The listing builds one solid part. Answer for the finished solid, in the listing's coordinates (mm). A direction names the side the tool comes from. Give positions to 0.01 mm unless a question says otherwise; leave off trailing zeros. Order: outer loops, then holes, each group sorted by start corner. A loop starts at its lowest first (then second) coordinate and runs counter-clockwise, first axis right, second up. Notation, with made-up numbers: (52, 75.25) - (67, 75.25) arc R36 cw to (67, 109.25) - close; hole circle Ø6 at (57, 56). An arc over 180 degrees is marked (long way). Use a Markdown table: item, result. Add a question column.
1) Flat-ended cylindrical pins translate along their axes: pin 1 (0.6 mm diameter, centred on y = -12, z = 1, fed in from -X); pin 2 (2 mm diameter, centred on x = 0, z = 2, fed in from +Y); pin 3 (1.9 mm diameter, centred on y = 16, z = -1.5, fed in from +X); pin 4 (4 mm diameter, centred on y = -8, z = 0, fed in from -X). Find the tip coordinate at first contact, or state that the pin passes through.
2) Find section A-A, the plane y = 8. Determine the outline of the cut face in (x, z).
3) Find section C-C, the plane z = 0. State how many separate pieces and enclosed holes the cut face has, plus the area to 3 significant figures.
4) Find section B-B, the plane x = 0.4. Determine the outline of the cut face in (y, z), plus the area to 3 significant figures.
5) Straight lines are drawn through the part: line 1 (Y direction, x = -0.45, z = 0); line 2 (Y direction, x = 0.65, z = 2); line 3 (X direction, y = -11.5, z = -2). For each, find the intervals that lie inside material, in ascending order.
6) For faces 3 (the face through (-1.606, -12.876, 0.694)), 4 (the face through (1.606, 4.876, 0.694)), 5 (the face through (0.017, 1.29, 2.024)), determine the directions among +Z, -Z, +X, -X, +Y, -Y from which every point of the face is accessible in a straight line to the end or side of a thin tool.
7) The mould has two halves that part along Y. Classify faces 1 (the face through (-2, -2, -3)), 2 (the face through (-1.2, 12, 0)): released by +Y, released by -Y, zero draft, split by the parting line, or undercut.
8) Find section D-D, the plane y = -10. Determine the outline of the cut face in (x, z).
Autodesk Inventor part; units mm, degrees
ref_plane "YZ Plane" through (0, 0, 0) normal (1, 0, 0) x (0, 1, 0)
ref_plane "XZ Plane" through (0, 0, 0) normal (0, 1, 0) x (-1, 0, 0)
ref_plane "XY Plane" through (0, 0, 0) normal (0, 0, 1) x (1, 0, 0)
sketch "Sketch3" plane through (0, 0, 0) normal (1, 0, 0) x (0, 1, 0)
  arc A0 (16, -3.6) -> (16, 3.6) centre (16, 0) ccw
  line L0 (-16, -3.6) -> (16, -3.6)
  line L1 (-16, 3.6) -> (16, 3.6)
  arc A1 (-16, 3.6) -> (-16, -3.6) centre (-16, 0) ccw
  line L2 (0, -3.6) -> (0, 3.6) construction
  circle A2 centre (-8, 0) radius 3.2
  circle A3 centre (0, 0) radius 3.2
  line L3 (0, 0) -> (-8, 0) construction
  line L4 (-8, 0) -> (-16, 0) construction
  circle A4 centre (-8, 0) radius 2.4
  circle A5 centre (0, 0) radius 2.4
  circle A6 centre (-16, 0) radius 3.2
  circle A7 centre (-16, 0) radius 2.4
  circle A8 centre (8, 0) radius 3.2
  circle A9 centre (8, 0) radius 2.4
  circle A10 centre (16, 0) radius 3.2
  circle A11 centre (16, 0) radius 2.4
  line L5 (0, 0) -> (8, 0) construction
  line L6 (8, 0) -> (16, 0) construction
  dimension "d49" = 7.2
  dimension "d59" = 6.4
  dimension "d60" = 4.8
  dimension "d64" = 8
extrude "Extrusion4" add sketch "Sketch3" along normal mid plane 4 contours L0 A1 L1 A0 | A2 | A3 | A6 | A8 | A10
sketch "Sketch11" plane through (2, 0, 0) normal (1, 0, 0) x (0, 0, -1)
  circle A0 centre (0, 0) radius 2.4
  circle A1 centre (0, -8) radius 2.4
  circle A2 centre (0, 0) radius 3.2
  circle A3 centre (0, -8) radius 3.2
  circle A4 centre (0, 8) radius 2.4
  arc A5 (3.6, 16) -> (-3.6, 16) centre (0, 16) ccw
  arc A6 (-3.6, -16) -> (3.6, -16) centre (0, -16) ccw
  circle A7 centre (0, -16) radius 3.2
  circle A8 centre (0, 8) radius 3.2
  circle A9 centre (0, 16) radius 3.2
  circle A10 centre (0, 16) radius 2.4
  line L0 (3.6, 16) -> (3.6, -16)
  line L1 (-3.6, -16) -> (-3.6, 16)
  line L2 (-2.5456, 13.4544) -> (-2.5456, 10.5456)
  line L3 (2.5456, 13.4544) -> (2.5456, 10.5456)
  arc A11 (-2.5456, 13.4544) -> (2.5456, 13.4544) centre (0, 16) ccw
  arc A12 (2.5456, 10.5456) -> (-2.5456, 10.5456) centre (0, 8) ccw
  line L4 (0, 16) -> (-2.5456, 13.4544) construction
  line L5 (-2.5456, 5.4544) -> (-2.5456, 2.5456)
  line L6 (2.5456, 5.4544) -> (2.5456, 2.5456)
  arc A13 (-2.5456, 5.4544) -> (2.5456, 5.4544) centre (0, 8) ccw
  arc A14 (2.5456, 2.5456) -> (-2.5456, 2.5456) centre (0, 0) ccw
  line L7 (-2.5456, -2.5456) -> (-2.5456, -5.4544)
  line L8 (2.5456, -2.5456) -> (2.5456, -5.4544)
  arc A15 (-2.5456, -2.5456) -> (2.5456, -2.5456) centre (0, 0) ccw
  arc A16 (2.5456, -5.4544) -> (-2.5456, -5.4544) centre (0, -8) ccw
  line L9 (-2.5456, -10.5456) -> (-2.5456, -13.4544)
  line L10 (2.5456, -10.5456) -> (2.5456, -13.4544)
  arc A17 (-2.5456, -10.5456) -> (2.5456, -10.5456) centre (0, -8) ccw
  arc A18 (2.5456, -13.4544) -> (-2.5456, -13.4544) centre (0, -16) ccw
  dimension "d61" = 6.4
  dimension "d65" = 45
  dimension "d68" = 8
extrude "Extrusion16" cut sketch "Sketch11" against normal blind 0.8 contours A0 | A1 | A2 | A3 | A4 | A7 | A8 | A9 | A10
extrude "Extrusion17" cut sketch "Sketch11" against normal blind 0.8 contours A11 L3 A12 L2 | A13 L6 A14 L5 | A15 L8 A16 L7 | A17 L10 A18 L9
mirror "Mirror3" about plane through (0, 0, 0) normal (1, 0, 0) of "Extrusion16", "Extrusion17"
fillet "Fillet1" radius 0.1 6 edges at (-2, 19.6, 0) (-2, 0, 3.6) (-2, 0, -3.6) (2, 0, 3.6) (2, 0, -3.6) (2, 19.6, 0)
fillet "Fillet1" radius 0.4 32 edges at (1.6, -13.4544, -2.5456) (1.6, -10.5456, -2.5456) (1.6, -10.5456, 2.5456) (1.6, -13.4544, 2.5456) (1.6, -5.4544, 2.5456) (1.6, -2.5456, 2.5456) (1.6, -2.5456, -2.5456) (1.6, -5.4544, -2.5456) (1.6, 2.5456, 2.5456) (1.6, 5.4544, 2.5456) (1.6, 5.4544, -2.5456) (1.6, 2.5456, -2.5456) (1.6, 10.5456, 2.5456) (1.6, 13.4544, 2.5456) (1.6, 13.4544, -2.5456) (1.6, 10.5456, -2.5456) (-1.6, -10.5456, -2.5456) (-1.6, -13.4544, -2.5456) (-1.6, -10.5456, 2.5456) (-1.6, -13.4544, 2.5456) (-1.6, -2.5456, 2.5456) (-1.6, -5.4544, 2.5456) (-1.6, -5.4544, -2.5456) (-1.6, -2.5456, -2.5456) (-1.6, 2.5456, -2.5456) (-1.6, 5.4544, -2.5456) (-1.6, 5.4544, 2.5456) (-1.6, 2.5456, 2.5456) (-1.6, 13.4544, 2.5456) (-1.6, 10.5456, 2.5456) (-1.6, 13.4544, -2.5456) (-1.6, 10.5456, -2.5456)
equation "\"d49\" = tlad"
equation "\"d59\" = tsd"
equation "\"d60\" = tpd"
equation "\"d64\" = lu"
equation "\"d15\" = 0.5 * lu"
equation "\"d61\" = tsd"
equation "\"d68\" = lu"
equation "\"d62\" = tsl"
equation "\"d73\" = 0.5 * lu - 2 * wall"
equation "\"d56\" = lf"
equation "\"d75\" = tf"
properties part number "32017-DKBluishGray" material "ABS Plastic"
The answers:
| question | item | result |
|---|---|---|
| 1 | pin 1 | x = -1.2 |
| 1 | pin 2 | y = 19.46 |
| 1 | pin 3 | x = 1.2 |
| 1 | pin 4 | through |
| 2 | outline | (-2, -3.5) arc R0.1 ccw to (-1.9, -3.6) - (1.9, -3.6) arc R0.1 ccw to (2, -3.5) - (2, -3.2) - (1.2, -3.2) - (1.2, -2.4) - (-1.2, -2.4) - (-1.2, -3.2) - (-2, -3.2) - close; (-2, 3.2) - (-1.2, 3.2) - (-1.2, 2.4) - (1.2, 2.4) - (1.2, 3.2) - (2, 3.2) - (2, 3.5) arc R0.1 ccw to (1.9, 3.6) - (-1.9, 3.6) arc R0.1 ccw to (-2, 3.5) - close |
| 3 | separate pieces | 6 |
| 3 | enclosed holes | 0 |
| 3 | area | 42.9 mm2 |
| 4 | outline | (-16, -3.6) - (16, -3.6) arc R3.6 ccw to (16, 3.6) - (-16, 3.6) arc R3.6 ccw to start; hole circle Ø4.8 at (-16, 0); hole circle Ø4.8 at (-8, 0); hole circle Ø4.8 at (0, 0); hole circle Ø4.8 at (8, 0); hole circle Ø4.8 at (16, 0) |
| 4 | area | 181 mm2 |
| 5 | line 1 | -19.6 to -18.4, -13.6 to -10.4, -5.6 to -2.4, 2.4 to 5.6, 10.4 to 13.6, 18.4 to 19.6 |
| 5 | line 2 | -18.99 to -17.33, -14.67 to -9.33, -6.67 to -1.33, 1.33 to 6.67, 9.33 to 14.67, 17.33 to 18.99 |
| 5 | line 3 | -1.2 to 1.2 |
| 6 | face 3 | -X |
| 6 | face 4 | +X |
| 6 | face 5 | +X, -X |
| 7 | face 1 | zero draft |
| 7 | face 2 | undercut |
| 8 | outline | (-2, -3.5) arc R0.1 ccw to (-1.9, -3.6) - (1.9, -3.6) arc R0.1 ccw to (2, -3.5) - (2, -2.5) - (1.2, -2.5) - (1.2, -1.33) - (-1.2, -1.33) - (-1.2, -2.5) - (-2, -2.5) - close; (-2, 2.5) - (-1.2, 2.5) - (-1.2, 1.33) - (1.2, 1.33) - (1.2, 2.5) - (2, 2.5) - (2, 3.5) arc R0.1 ccw to (1.9, 3.6) - (-1.9, 3.6) arc R0.1 ccw to (-2, 3.5) - close |
